from build123d import *

# Parameters (mm, degrees)
F0_W     = 100
F0_H     = 70
F0_R     = 2.25
F0_R_2   = 2.1
F1_DEPTH = 3


# Not quite as in the source:
# - a feature names something its author has since deleted; it is built from what else it names


with BuildPart() as f1:
    # F0 (on Top) → F1 (new body)
    with BuildSketch(Plane.XY):
        with Locations((-7.451e-07, 0.0999978185)):
            Rectangle(F0_W, F0_H)
        with Locations((-40.0000007451, -24.9000021815)):
            Circle(F0_R, mode=Mode.SUBTRACT)
        with Locations((40.0000007451, -24.9000021815)):
            Circle(F0_R, mode=Mode.SUBTRACT)
        Circle(F0_R_2, mode=Mode.SUBTRACT)
        with Locations((-40.0000007451, 25.0999978185)):
            Circle(F0_R, mode=Mode.SUBTRACT)
        with Locations((40.0000007451, 25.0999978185)):
            Circle(F0_R, mode=Mode.SUBTRACT)
    extrude(amount=F1_DEPTH)


solid = f1.part
Can you work these out from the model? Positions are in its coordinate system, mm. Give positions to 0.01 mm unless a question says otherwise; leave off trailing zeros. Write each loop counter-clockwise with the first axis right and the second up, starting at its lowest first coordinate (ties: lowest second). Pieces come first, ordered by that corner, then holes. Notation, with made-up numbers: (52.5, -33) -> (75.5, -33) arc R6 cw to (75.5, -24) -> close; hole circle Ø8 at (34.5, -19.5). An arc over 180 degrees is marked (long way). Answer as a JSON object with one key per item and string values. Group by question number.
Item 1: We'd pull the mould along Y, two halves only. Please class faces 1 (the face through (38.214, 23.731, 1.479)), 2 (the face through (-1, -34.9, 1)), 3 (the face through (-1, 8, 0)), 4 (the face through (-37.92, -25.76, 1.48)): +Y half, -Y half, draft (parallel to the pull), parting line (faces both ways), or undercut.
Item 2: Please list where these lines run through material, in increasing order: line 1 (Y direction, x = -40, z = 1.8); line 2 (Y direction, x = 0, z = 1); line 3 (Y direction, x = 39, z = 2.2). Write a range as [from, to].
Item 3: Suppose I cut it at B-B (x = 0). Please give me the cut outline in (y, z).
Item 4: Suppose I cut it at A-A (x = -40). Please give me the cut outline in (y, z).
Item 5: Suppose I cut it at C-C (y = 0). Please give me the cut outline in (x, z), plus the area to 3 significant figures.
Findings:
{
 "1": {"face 1": "undercut", "face 2": "-Y half", "face 3": "draft", "face 4": "undercut"},
 "2": {"line 1": "y = [-34.9, -27.15], [-22.65, 22.85], [27.35, 35.1]", "line 2": "y = [-34.9, -2.1], [2.1, 35.1]", "line 3": "y = [-34.9, -26.92], [-22.88, 23.08], [27.12, 35.1]"},
 "3": {"outline": "(-34.9, 0) -> (-2.1, 0) -> (-2.1, 3) -> (-34.9, 3) -> close; (2.1, 0) -> (35.1, 0) -> (35.1, 3) -> (2.1, 3) -> close"},
 "4": {"outline": "(-34.9, 0) -> (-27.15, 0) -> (-27.15, 3) -> (-34.9, 3) -> close; (-22.65, 0) -> (22.85, 0) -> (22.85, 3) -> (-22.65, 3) -> close; (27.35, 0) -> (35.1, 0) -> (35.1, 3) -> (27.35, 3) -> close"},
 "5": {"outline": "(-50, 0) -> (-2.1, 0) -> (-2.1, 3) -> (-50, 3) -> close; (2.1, 0) -> (50, 0) -> (50, 3) -> (2.1, 3) -> close", "area": "287 mm²"}
}
